Read the model definition and answer for the solid it produces. Units are mm, in the model's axes. A direction names the side the tool comes from. Round coordinates to 2 decimals unless told otherwise and drop trailing zeros. Loops run counter-clockwise (first coordinate to the right, second up) from the corner with the lowest first, then second, coordinate; pieces in that order, holes last. Notation, with made-up numbers: M 87.5,14.5 L 130.5,14.5 A35 ccw 130.5,47.5 Z; hole C 60.5,86 d7. An arc over 180 degrees is marked long. Write each question's results on one line, items separated by ' | '.
```python
from build123d import *

# Parameters (mm, degrees)
F1_DEPTH = 0.2032
F2_SCALE = 12


with BuildPart() as f1:
    # F0 (on Right) → F1 (new body, symmetric)
    with BuildSketch(Plane.YZ):
        with BuildLine():
            ThreePointArc((7.6535586268, -3.8887472606), (7.7279535043, -4.0683523831), (7.9075586268, -4.1427472606))
            Line((7.9075586268, -4.1427472606), (58.4309190295, -4.1427472606))
            ThreePointArc((58.4309190295, -4.1427472606), (58.6105241519, -4.0683523831), (58.6849190295, -3.8887472606))
            Line((58.6849190295, -3.8887472606), (58.6849190295, 21.1963314346))
            ThreePointArc((58.6849190295, 21.1963314346), (58.6105241519, 21.375936557), (58.4309190295, 21.4503314346))
            Line((58.4309190295, 21.4503314346), (7.9075586268, 21.4503314346))
            ThreePointArc((7.9075586268, 21.4503314346), (7.7279535043, 21.375936557), (7.6535586268, 21.1963314346))
            Line((7.6535586268, 21.1963314346), (7.6535586268, -3.8887472606))
        make_face()
        with BuildLine():
            ThreePointArc((32.8605727571, 4.9196215098), (32.5678123501, 5.0882773482), (32.7015852855, 5.3985324844))
            Line((32.7015852855, 5.3985324844), (56.9304593399, 16.6896579893))
            ThreePointArc((56.9304593399, 16.6896579893), (57.1742493276, 16.6736356668), (57.2917498648, 16.4594303992))
            Line((57.2917498648, 16.4594303992), (57.2917498648, 10.2050660498))
            ThreePointArc((57.2917498648, 10.2050660498), (57.2347866945, 10.0447772861), (57.0894468115, 9.9563826653))
            Line((57.0894468115, 9.9563826653), (32.8605727571, 4.9196215098))
        make_face(mode=Mode.SUBTRACT)
    extrude(amount=F1_DEPTH, both=True)


with BuildPart() as f1_1:
    # F2: moved
    add(f1.part.scale(F2_SCALE))


solid = f1_1.part
```
1. Find section C-C, the plane z = 182. Give the vertices of the cut face in (x, y), then the cut area to 3 significant figures.
Completed:
outline: M -2.44,91.84 L 2.44,91.84 L 2.44,643.95 L -2.44,643.95 Z; M -2.44,687.5 L 2.44,687.5 L 2.44,704.22 L -2.44,704.22 Z | area: 2,770 mm2
2. Find section B-B, the plane x = 1. Give the vertices of the cut face in (y, z), then the cut area to 3 significant figures.
Completed:
outline: M 91.84,-46.66 A3.05 ccw 94.89,-49.71 L 701.17,-49.71 A3.05 ccw 704.22,-46.66 L 704.22,254.36 A3.05 ccw 701.17,257.4 L 94.89,257.4 A3.05 ccw 91.84,254.36 Z; hole M 392.42,64.78 A3.05 ccw 394.33,59.04 L 685.07,119.48 A3.05 ccw 687.5,122.46 L 687.5,197.51 A3.05 ccw 683.17,200.28 Z | area: 175,000 mm2
3. Determine the mould class of faces 3 (the face through (0, 535.8, 131.6)), 4 (the face through (2.438, 394, 106)) for opening direction Y: released by +Y, released by -Y, zero draft, split by the parting line, or undercut.
Completed:
face 3: undercut | face 4: zero draft
4. Find section A-A, the plane y = 639. Give the vertices of the cut face in (x, z).
Completed:
outline: M -2.44,-49.71 L 2.44,-49.71 L 2.44,109.9 L -2.44,109.9 Z; M -2.44,179.69 L 2.44,179.69 L 2.44,257.4 L -2.44,257.4 Z
5. Which of the six approach directions +Z, -Z, +X, -X, +Y, -Y give full straight-line access (tool end or side, diameter ignored) to faces 1 (the face through (0.03, 541.74, 89.68)), 2 (the face through (-2.438, 394, 106))?
Completed:
face 1: +X, -X | face 2: +Z, -Z, -X, +Y, -Y
6. Find the intervals of material crossed by L1, parallel to Z at x = -0.2, y = 590.5; L2, parallel to Z at x = -1.95, y = 442; L3, parallel to Y at x = 0.2, z = 126, in increasing order.
Completed:
L1: z = -49.71 to 99.82, 157.09 to 257.4 | L2: z = -49.71 to 68.95, 87.89 to 257.4 | L3: y = 91.84 to 523.78, 687.5 to 704.22
